```python
from build123d import *

# Parameters (mm, degrees)
BOSS_EXTRUDE1_DEPTH = 9
SKETCH10_W          = 31
SKETCH10_H          = 17
BOSS_EXTRUDE5_DEPTH = 59
SKETCH11_R          = 1.75
SKETCH11_W          = 21
SKETCH11_H          = 41
CUT_EXTRUDE6_DEPTH  = 38
SKETCH12_R          = 1.75
CUT_EXTRUDE7_DEPTH  = 3


with BuildPart() as part:
    # Sketch1 → Boss-Extrude1 (new body)
    with BuildSketch(Plane.XY):
        Polygon((15.5, -28.5), (-15.5, -28.5), (-15.5, -10.3), (-15.5, 10.3), (-15.5, 28.5), (15.5, 28.5), align=None)
    extrude(amount=BOSS_EXTRUDE1_DEPTH)

    # Sketch10 → Boss-Extrude5 (add)
    with BuildSketch(Plane.XY.offset(9)):
        Rectangle(SKETCH10_W, SKETCH10_H)
    extrude(amount=BOSS_EXTRUDE5_DEPTH)

    # Sketch11 → Cut-Extrude6 (cut, through all)
    with BuildSketch(Plane.XZ.offset(8.5)):
        with Locations((5.2, 13.5)):
            Circle(SKETCH11_R)
        with Locations((-5.2, 13.5)):
            Circle(SKETCH11_R)
        with Locations((5.2, 63.5)):
            Circle(SKETCH11_R)
        with Locations((-5.2, 63.5)):
            Circle(SKETCH11_R)
        with Locations((0, 38.5)):
            Rectangle(SKETCH11_W, SKETCH11_H)
    extrude(amount=-CUT_EXTRUDE6_DEPTH, mode=Mode.SUBTRACT)

    # Sketch12 → Cut-Extrude7 (cut)
    with BuildSketch(Plane(origin=(0, 0, 0), x_dir=(-1, 0, 0), z_dir=(0, 0, -1))):
        with Locations((11.5, 25)):
            Circle(SKETCH12_R)
        with Locations((-11.5, 25)):
            Circle(SKETCH12_R)
        with Locations((11.5, -25)):
            Circle(SKETCH12_R)
        with Locations((-11.5, -25)):
            Circle(SKETCH12_R)
    extrude(amount=-CUT_EXTRUDE7_DEPTH, mode=Mode.SUBTRACT)


solid = part.part
```
The listing builds one solid part. Answer for the finished solid, in the listing's coordinates (mm). A direction names the side the tool comes from. Give positions to 0.01 mm unless a question says otherwise; leave off trailing zeros. Order: outer loops, then holes, each group sorted by start corner. A loop starts at its lowest first (then second) coordinate and runs counter-clockwise, first axis right, second up. Notation, with made-up numbers: (54, -12) -> (79, -12) arc R18 ccw to (79, 21) -> close; hole circle Ø8 at (74.5, -38). An arc over 180 degrees is marked (long way). Write each question's results on one line, items separated by ' | '.
Q1. Which of the six approach directions +Z, -Z, +X, -X, +Y, -Y give full straight-line access (tool end or side, diameter ignored) to faces 1 (the face through (12, 25, 3)), 2 (the face through (0, 0, 68)), 3 (the face through (-11, 8.5, 38)), 4 (the face through (-11, -8.5, 38)), 5 (the face through (0, 0, 18))?
Checked values:
face 1: -Z | face 2: +Z, +X, -X, +Y, -Y | face 3: +Z, +X, -X, +Y | face 4: +Z, +X, -X, -Y | face 5: +Y, -Y
Q2. Each of these flat-tipped pins is pushed along its axis until it touches: P1, Ø10, axis at x = 5, y = 6.5, coming from the -Z side; P2, Ø5.5, axis at x = 5.2, z = 63.5, coming from the -Y side; P3, Ø3, axis at y = 11, z = 45.5, coming from the -X side; P4, Ø3, axis at x = -11.5, y = -25, coming from the +Z side. Where does it stop, or does it pass through?
Checked values:
P1: stops at z = 0 | P2: stops at y = -8.5 | P3: passes through | P4: stops at z = 9
Q3. The part is cut by section D-D, the plane z = 20.5. Give the vertices of the cut face in (x, y).
Checked values:
outline: (-15.5, -8.5) -> (-10.5, -8.5) -> (-10.5, 8.5) -> (-15.5, 8.5) -> close; (10.5, -8.5) -> (15.5, -8.5) -> (15.5, 8.5) -> (10.5, 8.5) -> close
Q4. The part is cut by section A-A, the plane y = 1. Give the vertices of the cut face in (x, z), and give its area (3 significant figures).
Checked values:
outline: (-15.5, 0) -> (15.5, 0) -> (15.5, 68) -> (-15.5, 68) -> close; hole (-10.5, 18) -> (10.5, 18) -> (10.5, 59) -> (-10.5, 59) -> close; hole circle Ø3.5 at (-5.2, 13.5); hole circle Ø3.5 at (-5.2, 63.5); hole circle Ø3.5 at (5.2, 13.5); hole circle Ø3.5 at (5.2, 63.5) | area: 1,210 mm^2
Q5. Straight lines are drawn through the part: probe 1 along Z at (x, y) = (-5, -1); probe 2 along Y at (x, z) = (-11.5, 0.65); probe 3 along Z at (x, y) = (-7.5, 6). For each, find the intervals that lie inside material, in ascending order. Write a range as from..to.
Checked values:
probe 1: z = 0..11.76, 15.24..18, 59..61.76, 65.24..68 | probe 2: y = -28.5..-26.75, -23.25..23.25, 26.75..28.5 | probe 3: z = 0..18, 59..68
Q6. Determine the mould class of faces 6 (the face through (11.728, 26.735, 1.479)), 7 (the face through (12, -25, 3)), 8 (the face through (4.82, -0.12, 61.79)) for opening direction Z: pulls with the +Z half, pulls with the -Z half, needs draft (parallel to the pull), parting line crosses it, or undercut.
Checked values:
face 6: needs draft | face 7: pulls with the -Z half | face 8: undercut
Q7. The part is cut by section C-C, the plane x = -6. Give the vertices of the cut face in (y, z).
Checked values:
outline: (-28.5, 0) -> (28.5, 0) -> (28.5, 9) -> (8.5, 9) -> (8.5, 11.94) -> (-8.5, 11.94) -> (-8.5, 9) -> (-28.5, 9) -> close; (-8.5, 15.06) -> (8.5, 15.06) -> (8.5, 18) -> (-8.5, 18) -> close; (-8.5, 59) -> (8.5, 59) -> (8.5, 61.94) -> (-8.5, 61.94) -> close; (-8.5, 65.06) -> (8.5, 65.06) -> (8.5, 68) -> (-8.5, 68) -> close
Q8. The part is cut by section B-B, the plane z = 13.5. Give the vertices of the cut face in (x, y).
Checked values:
outline: (-15.5, -8.5) -> (-6.95, -8.5) -> (-6.95, 8.5) -> (-15.5, 8.5) -> close; (-3.45, -8.5) -> (3.45, -8.5) -> (3.45, 8.5) -> (-3.45, 8.5) -> close; (6.95, -8.5) -> (15.5, -8.5) -> (15.5, 8.5) -> (6.95, 8.5) -> close
